Model file for the job. Use its own axes, mm. Face numbers are marked on the shaded views. A direction names the side the tool comes from. Give positions to 0.01 mm unless a question says otherwise; leave off trailing zeros. Order: outer loops, then holes, each group sorted by start corner. A loop starts at its lowest first (then second) coordinate and runs counter-clockwise, first axis right, second up. Notation, with made-up numbers: M -26,40.25 L 2,40.25 A28 cw 2,64.25 Z; hole C 79.5,68 d7. An arc over 180 degrees is marked long. Return JSON: item names as keys, results as strings. Group by question number.
1. Slice it at A-A on x = 15.24. List the corners of the cut face in (y, z).
2. Pin check, flat tips, straight feed: pin 1 (14 mm diameter, centred on x = 12.5, z = 11, fed in from -Y); pin 2 (5 mm diameter, centred on x = 14, z = 22.5, fed in from -Y); pin 3 (3 mm diameter, centred on x = 29.5, y = 22, fed in from +Z); pin 4 (1.3 mm diameter, centred on x = 1.5, y = 17, fed in from -Z). Stop position of each tip, or through.
3. Wall check: probe 1 along Z at (x, y) = (15.24, 74.3); probe 2 along X at (y, z) = (4, 0.5); probe 3 along X at (y, z) = (75, -25). Give the ranges that are in metal, low to high. Write a range as [from, to].
4. Slice it at B-B on x = 25. List the corners of the cut face in (y, z).
5. Slice it at D-D on y = 30. List the corners of the cut face in (x, z), then the cut area to 3 significant figures.
6. Slice it at C-C on z = 28. List the corners of the cut face in (x, y).
7. 3-axis set-ups, long thin cutter, end or side, ignore diameter. For the marked faces 1, 2 and 3: which of +Z, -Z, +X, -X, +Y, -Y reach the whole face in a straight line?
8. Two-plate mould, pull along X, no slides. Class the marked faces 4, 5 and 6: released by +X, released by -X, zero draft, split by the parting line, or undercut.
from build123d import *

# Parameters (mm, degrees)
BOSS_EXTRUDE1_DEPTH     = 50.8
SKETCH4_W               = 25.4
SKETCH4_H               = 45.212
CUT_EXTRUDE1_DEPTH      = 1
CUT_EXTRUDE1_DEPTH_BACK = 31.48
CUT_EXTRUDE4_DEPTH      = 1
CUT_EXTRUDE4_DEPTH_BACK = 31.48
SKETCH8_R               = 6.35
BOLT_HOLES_DEPTH        = 1
BOLT_HOLES_DEPTH_BACK   = 77.2
FILLET3_R               = 12.7
FILLET4_R               = 1.5875


with BuildPart() as part:
    # Sketch1 → Boss-Extrude1 (new body, symmetric)
    with BuildSketch(Plane.XY):
        Polygon((0, 76.2), (30.48, 76.2), (30.48, 73.66), (30.48, 47.752), (30.48, 0), (27.94, 0), (27.94, 45.212), (2.54, 45.212), (2.54, 0), (0, 0), (0, 47.752), (27.94, 47.752), (27.94, 73.66), (0, 73.66), align=None)
    extrude(amount=BOSS_EXTRUDE1_DEPTH, both=True)

    # Sketch4 → Cut-Extrude1 (cut, two sides)
    with BuildSketch(Plane(origin=(30.48, 0, 0), x_dir=(0, 0, -1), z_dir=(1, 0, 0))) as cut_extrude1_sk:
        with Locations((-38.1, 22.606)):
            Rectangle(SKETCH4_W, SKETCH4_H)
        with Locations((38.1, 22.606)):
            Rectangle(SKETCH4_W, SKETCH4_H)
    extrude(amount=CUT_EXTRUDE1_DEPTH, mode=Mode.SUBTRACT)
    extrude(cut_extrude1_sk.sketch, amount=-CUT_EXTRUDE1_DEPTH_BACK, mode=Mode.SUBTRACT)

    # Sketch7 → Cut-Extrude4 (cut, two sides)
    with BuildSketch(Plane(origin=(30.48, 0, 0), x_dir=(0, 0, -1), z_dir=(1, 0, 0))) as cut_extrude4_sk:
        with BuildLine():
            Line((-2.079997498, 26.98812083), (25.4, 35.56))
            Line((25.4, 35.56), (25.4, 20.926124507))
            Line((25.4, 20.926124507), (2.079997498, 13.65187917))
            ThreePointArc((2.079997498, 13.65187917), (-6.66812083, 18.240002502), (-2.079997498, 26.98812083))
        make_face()
    extrude(amount=CUT_EXTRUDE4_DEPTH, mode=Mode.SUBTRACT)
    extrude(cut_extrude4_sk.sketch, amount=-CUT_EXTRUDE4_DEPTH_BACK, mode=Mode.SUBTRACT)

    # Sketch8 → BOLT HOLES (cut, two sides)
    with BuildSketch(Plane(origin=(0, 76.2, 0), x_dir=(1, 0, 0), z_dir=(0, 1, 0))) as bolt_holes_sk:
        with Locations((15.24, -25.4)):
            Circle(SKETCH8_R)
        with Locations((15.24, 25.4)):
            Circle(SKETCH8_R)
    extrude(amount=BOLT_HOLES_DEPTH, mode=Mode.SUBTRACT)
    extrude(bolt_holes_sk.sketch, amount=-BOLT_HOLES_DEPTH_BACK, mode=Mode.SUBTRACT)

    # Fillet3
    fillet3_edges = [part.edges().sort_by_distance(p)[0] for p in [
        (1.27, 0, 25.4),
        (29.21, 0, 25.4),
        (1.27, 0, -25.4),
        (29.21, 0, -25.4),
    ]]
    fillet(fillet3_edges, radius=FILLET3_R)

    # Fillet4
    fillet4_edges = [part.edges().sort_by_distance(p)[0] for p in [
        (1.27, 35.56, -25.4),
        (29.21, 35.56, -25.4),
        (1.27, 20.926124507, -25.4),
        (29.21, 20.926124507, -25.4),
    ]]
    fillet(fillet4_edges, radius=FILLET4_R)


solid = part.part
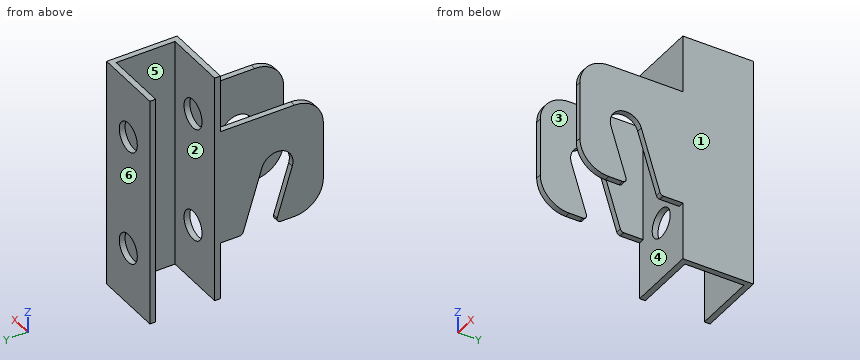
Result:
{
 "1": {"outline": "M 45.21,-50.8 L 47.75,-50.8 L 47.75,-31.75 L 45.21,-31.75 Z; M 45.21,-19.05 L 47.75,-19.05 L 47.75,19.05 L 45.21,19.05 Z; M 45.21,31.75 L 47.75,31.75 L 47.75,50.8 L 45.21,50.8 Z; M 73.66,-50.8 L 76.2,-50.8 L 76.2,-31.75 L 73.66,-31.75 Z; M 73.66,-19.05 L 76.2,-19.05 L 76.2,19.05 L 73.66,19.05 Z; M 73.66,31.75 L 76.2,31.75 L 76.2,50.8 L 73.66,50.8 Z"},
 "2": {"pin 1": "stops at y = 45.21", "pin 2": "passes through", "pin 3": "stops at z = 25.4", "pin 4": "stops at z = -25.4"},
 "3": {"probe 1": "z = [-50.8, -31.75], [-19.05, 19.05], [31.75, 50.8]", "probe 2": "x = [0, 2.54], [27.94, 30.48]", "probe 3": "x = [0, 8.9], [21.58, 30.48]"},
 "4": {"outline": "M 45.21,-50.8 L 47.75,-50.8 L 47.75,50.8 L 45.21,50.8 Z; M 73.66,-50.8 L 76.2,-50.8 L 76.2,50.8 L 73.66,50.8 Z"},
 "5": {"outline": "M 0,-7.58 L 2.54,-7.58 L 2.54,25.4 L 0,25.4 Z; M 27.94,-7.58 L 30.48,-7.58 L 30.48,25.4 L 27.94,25.4 Z", "area": "168 mm2"},
 "6": {"outline": "M 0,45.21 L 9.45,45.21 L 9.45,47.75 L 0,47.75 Z; M 0,73.66 L 9.45,73.66 L 9.45,76.2 L 0,76.2 Z; M 21.03,45.21 L 30.48,45.21 L 30.48,76.2 L 21.03,76.2 L 21.03,73.66 L 27.94,73.66 L 27.94,47.75 L 21.03,47.75 Z"},
 "7": {"face 1": "+Z, -Z, +X, +Y, -Y", "face 2": "+Z, -Z, -X", "face 3": "+Z, -Z, -Y"},
 "8": {"face 4": "undercut", "face 5": "released by -X", "face 6": "zero draft"}
}
